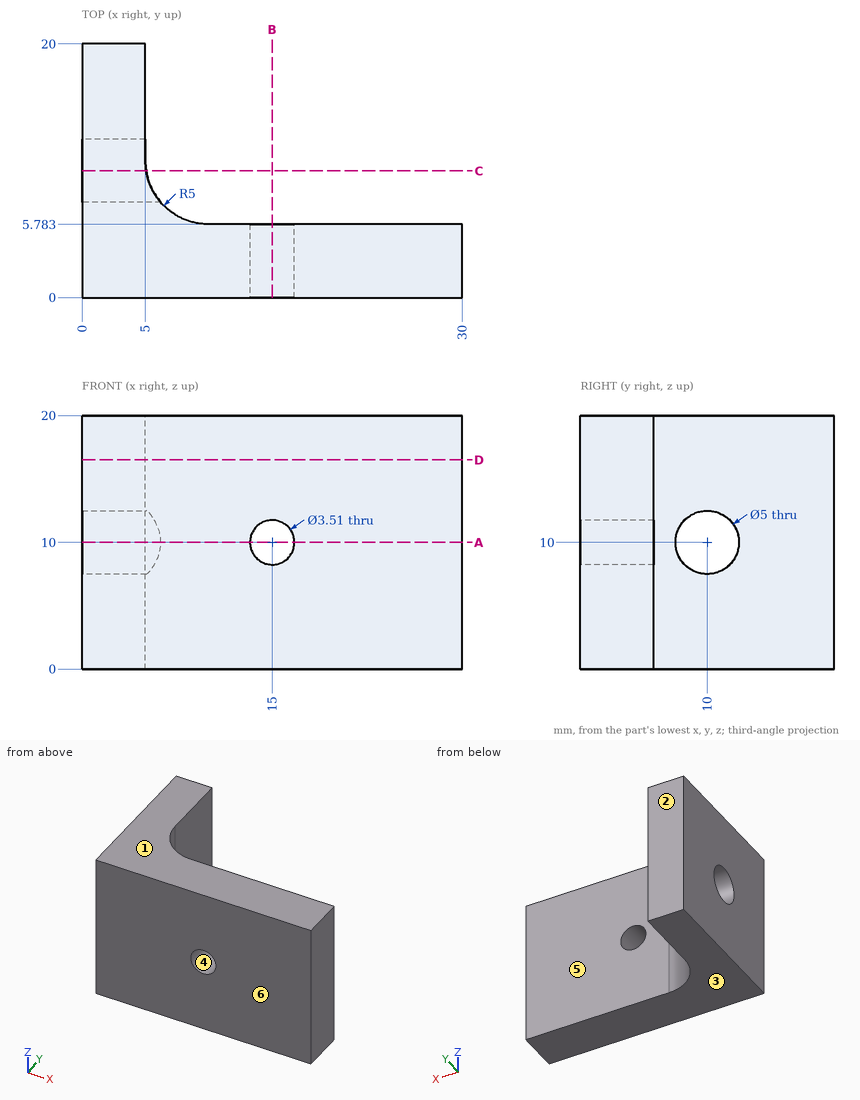
Drawing for the job (mm, zero at the part's lowest x, y, z). A direction names the side the tool comes from. Give positions to 0.01 mm unless a question says otherwise; leave off trailing zeros. Order: outer loops, then holes, each group sorted by start corner. A loop starts at its lowest first (then second) coordinate and runs counter-clockwise, first axis right, second up. Notation, with made-up numbers: M -6,27 L 50,27 A18 ccw 50,50 Z; hole C 70.5,31.5 d3. An arc over 180 degrees is marked long. Put each result on its own line as item: value.
Item 1: Slice it at A-A, the plane z = 10. Write the cut outline in (x, y) (3 decimals), plus the area to 3 significant figures.
From the geometry:
outline: M 0,0 L 13.245,0 L 13.245,5.783 L 10,5.783 A5 cw 6.229,7.5 L 0,7.5 Z; M 0,12.5 L 5,12.5 L 5,20 L 0,20 Z; M 16.755,0 L 30,0 L 30,5.783 L 16.755,5.783 Z
area: 203 mm2
Item 2: Flat gauge pins, fed straight in: pin 1 Ø1.5 at (x, z) = (17, 5.5) entering from +Y; pin 2 Ø2 at (y, z) = (18, 14.5) entering from +X; pin 3 Ø2 at (x, z) = (14, 15) entering from -Y; pin 4 Ø4 at (x, z) = (9, 3.5) entering from +Y. Where does each tip first touch, or does it go through?
From the geometry:
pin 1: stops at y = 5.78
pin 2: stops at x = 5
pin 3: stops at y = 0
pin 4: stops at y = 6.78
Item 3: Slice it at B-B, the plane x = 15. Write the cut outline in (y, z) (3 decimals).
From the geometry:
outline: M 0,0 L 5.783,0 L 5.783,8.245 L 0,8.245 Z; M 0,11.755 L 5.783,11.755 L 5.783,20 L 0,20 Z
Item 4: Probe line 1 (Y direction, x = 3, z = 10); line 2 (Z direction, x = 15, y = 2.1) (3 decimals). List the from-to ranges inside material, lowest first. Write a range as [from, to].
From the geometry:
line 1: y = [0, 7.5], [12.5, 20]
line 2: z = [0, 8.245], [11.755, 20]
Item 5: Slice it at C-C, the plane y = 10. Write the cut outline in (x, z).
From the geometry:
outline: M 0,0 L 5.06,0 L 5.06,7.5 L 0,7.5 Z; M 0,12.5 L 5.06,12.5 L 5.06,20 L 0,20 Z
Item 6: 3-axis set-ups, long thin cutter, end or side, ignore diameter. For the marked faces 5 and 6: which of +Z, -Z, +X, -X, +Y, -Y reach the whole face in a straight line?
From the geometry:
face 5: +Z, -Z, +X, +Y
face 6: +Z, -Z, +X, -X, -Y
Item 7: Slice it at D-D, the plane z = 16.5. Write the cut outline in (x, y).
From the geometry:
outline: M 0,0 L 30,0 L 30,5.78 L 10,5.78 A5 cw 5,10.78 L 5,20 L 0,20 Z
Item 8: Two-plate mould, pull along Z, no slides. Class the marked faces 1, 2, 3 and 4: +Z half, -Z half, draft (parallel to the pull), parting line (faces both ways), or undercut.
From the geometry:
face 1: +Z half
face 2: draft
face 3: -Z half
face 4: undercut
